from build123d import *

# Parameters (mm, degrees)
F0_W     = 1000
F0_H     = 400
F1_DEPTH = 20
F2_W     = 50
F2_H     = 50
F3_DEPTH = 1000
F4_W     = 900
F4_H     = 20
F4_W_2   = 20
F4_H_2   = 300
F5_DEPTH = 100


with BuildPart() as f1:
    # F0 (on Top) → F1 (new body)
    with BuildSketch(Plane.XY):
        with Locations((-500, -200)):
            Rectangle(F0_W, F0_H)
    extrude(amount=-F1_DEPTH)

    # F2 (on face) → F3 (join)
    with BuildSketch(Plane(origin=(0, 0, -20), x_dir=(1, 0, 0), z_dir=(0, 0, -1))):
        with Locations((-25, 25)):
            Rectangle(F2_W, F2_H)
        with Locations((-975, 25)):
            Rectangle(F2_W, F2_H)
    extrude(amount=F3_DEPTH)

    # F4 (on face) → F5 (join)
    with BuildSketch(Plane(origin=(0, 0, -20), x_dir=(1, 0, 0), z_dir=(0, 0, -1))):
        with Locations((-500, 20)):
            Rectangle(F4_W, F4_H)
        with Locations((-20, 200)):
            Rectangle(F4_W_2, F4_H_2)
        with Locations((-980, 200)):
            Rectangle(F4_W_2, F4_H_2)
    extrude(amount=F5_DEPTH)


solid = f1.part
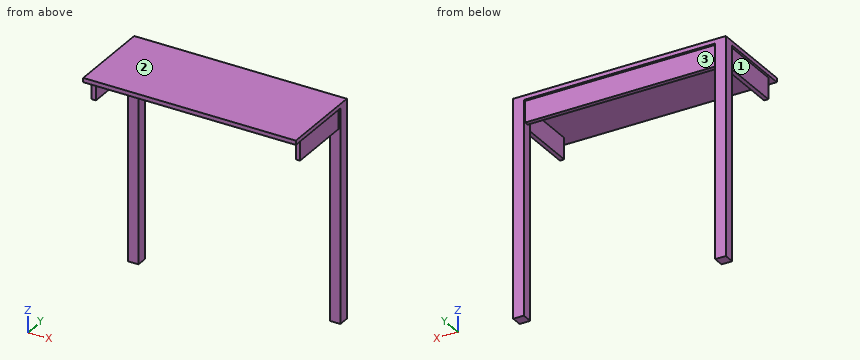
Design review of the part built by this model. Coordinates are the model's own, in mm. Face numbers are marked on the shaded views. Give positions to 0.01 mm unless a question says otherwise; leave off trailing zeros. Loops run counter-clockwise (first coordinate to the right, second up) from the corner with the lowest first, then second, coordinate; pieces in that order, holes last. Notation, with made-up numbers: (-7, 52) -> (14, 52) arc R30 cw to (14, 80) -> close; hole circle Ø1 at (47.5, 60). An arc over 180 degrees is marked (long way). One line per question, with ' | ' between items. Start each with the question number.
(1) For line 1 (X direction, y = -55.5, z = -104); line 2 (X direction, y = -25, z = -361); line 3 (Z direction, x = -467, y = -36.5), list the stretches that pass through material, from the lowest coordinate up.
(2) Draft analysis for pull direction X (two halves, no side actions). For the marked faces 1, 2 and 3, state which applies: +X half, -X half, draft (parallel to the pull), parting line (faces both ways), or undercut.
(3) We need section A-A (z = -632). State the section outline as (x, y) points, and give its area (3 significant figures).
(4) We need section B-B (x = -270). State the section outline as (y, z) points.
(5) Insertion check: P1, Ø16, axis at x = -19, z = -61.5, coming from the -Y side; P2, Ø8, axis at x = -559.5, y = -322, coming from the -Z side; P3, Ø10, axis at x = -977.5, y = -153, coming from the -Z side. Each pin has a flat end and moves straight along its axis. Give the tip position at first contact, or say it passes through.
(6) We need section C-C (y = -243). State the section outline as (x, z) points, and give its area (3 significant figures).
The answers:
1) line 1: x = -990 to -970, -30 to -10 | line 2: x = -1000 to -950, -50 to 0 | line 3: z = -20 to 0
2) face 1: -X half | face 2: draft | face 3: undercut
3) outline: (-1000, -50) -> (-950, -50) -> (-950, 0) -> (-1000, 0) -> close; (-50, -50) -> (0, -50) -> (0, 0) -> (-50, 0) -> close | area: 5,000 mm^2
4) outline: (-400, -20) -> (-30, -20) -> (-30, -120) -> (-10, -120) -> (-10, -20) -> (0, -20) -> (0, 0) -> (-400, 0) -> close
5) P1: stops at y = -350 | P2: stops at z = -20 | P3: stops at z = -120
6) outline: (-1000, -20) -> (-990, -20) -> (-990, -120) -> (-970, -120) -> (-970, -20) -> (-30, -20) -> (-30, -120) -> (-10, -120) -> (-10, -20) -> (0, -20) -> (0, 0) -> (-1000, 0) -> close | area: 24,000 mm^2
